Input: part model. Units: mm. Frame: model coordinates. A direction names the side the tool comes from. Give positions to 0.01 mm unless a question says otherwise; leave off trailing zeros. Order: outer loops, then holes, each group sorted by start corner. A loop starts at its lowest first (then second) coordinate and runs counter-clockwise, first axis right, second up. Notation, with made-up numbers: (32, -16.5) -> (52, -16.5) arc R29 cw to (52, 19.5) -> close; hole circle Ø3 at (6, -25). An arc over 180 degrees is marked (long way). Use a Markdown table: item, result. Add a question column.
from build123d import *

# Parameters (mm, degrees)
F1_R = 4.7625


with BuildPart() as f2:
    # F2: sweep along a path in F0
    with BuildLine(Plane.YZ) as f2_path:
        Line((0, 0), (0, 6.35))
        ThreePointArc((0, 6.35), (1.8598719395, 10.8401280605), (6.35, 12.7))
        Line((6.35, 12.7), (69.85, 12.7))
        ThreePointArc((69.85, 12.7), (74.3401280605, 10.8401280605), (76.2, 6.35))
        Line((76.2, 6.35), (76.2, 0))
    # F1 (on Top) → F2 (sweep)
    with BuildSketch(Plane.XY):
        Circle(F1_R)
    sweep(path=f2_path.line)


solid = f2.part
Q1. First-contact query: pin 1 (1 mm diameter, centred on x = -2, z = 12, fed in from -Y); pin 2 (1 mm diameter, centred on y = 40.5, z = 13.5, fed in from +X); pin 3 (1.5 mm diameter, centred on x = -2, y = 28, fed in from +Z); pin 4 (6 mm diameter, centred on y = 51.5, z = 2, fed in from +X). Flat tips, straight axial feed; report the tip coordinate or a pass-through.
Q2. Ray query, line 1 (Y direction, x = 0, z = 2); line 2 (Y direction, x = 4, z = 8.5); line 3 (Z direction, x = -0.25, y = 23). Return the intervals inside material, ascending.
Q3. Access query for faces 1 (the flat face through (0, 0, 0)), 2 (the cylindrical face through (3, 39, 9)), 3 (the cylindrical face through (-0.62, 71.48, 3.13)). Directions: +Z, -Z, +X, -X, +Y, -Y. A direction counts if a zero-diameter tool reaches every point of the face in a straight line with its end or side. Return the directions, or none.
Q4. Draft query along Y for faces 4 (the cylindrical face through (-3.78, -2.9, 3.22)), 5 (the flat face through (0, 76, 0)). Return one class per face: +Y half, -Y half, draft (parallel to the pull), parting line (faces both ways), or undercut.
Q5. Section query C-C (y = 17). Return loops of the section in (x, z) (1 decimal).
Q6. Section query B-B (z = 2.5). Return loops of the section in (x, y) (1 decimal).
Q7. Section query D-D (x = -3.25). Return loops of the section in (y, z), plus the area to 3 significant figures.
Solution:
| question | item | result |
|---|---|---|
| 1 | pin 1 | stops at y = -3.09 |
| 1 | pin 2 | stops at x = 4.75 |
| 1 | pin 3 | stops at z = 17.3 |
| 1 | pin 4 | passes through |
| 2 | line 1 | y = -4.76 to 4.76, 71.44 to 80.96 |
| 2 | line 2 | y = -2.32 to 3.26, 72.94 to 78.52 |
| 2 | line 3 | z = 7.94 to 17.46 |
| 3 | face 1 | -Z, +X, -X, +Y, -Y |
| 3 | face 2 | none |
| 3 | face 3 | -Z |
| 4 | face 4 | undercut |
| 4 | face 5 | draft |
| 5 | outline | circle Ø9.5 at (0, 12.7) |
| 6 | outline | circle Ø9.5 at (0, 0); circle Ø9.5 at (0, 76.2) |
| 7 | outline | (-3.48, 0) -> (3.48, 0) -> (3.48, 6.35) arc R2.87 cw to (6.35, 9.22) -> (69.85, 9.22) arc R2.87 cw to (72.72, 6.35) -> (72.72, 0) -> (79.68, 0) -> (79.68, 6.35) arc R9.83 ccw to (69.85, 16.18) -> (6.35, 16.18) arc R9.83 ccw to (-3.48, 6.35) -> close |
| 7 | area | 669 mm² |
